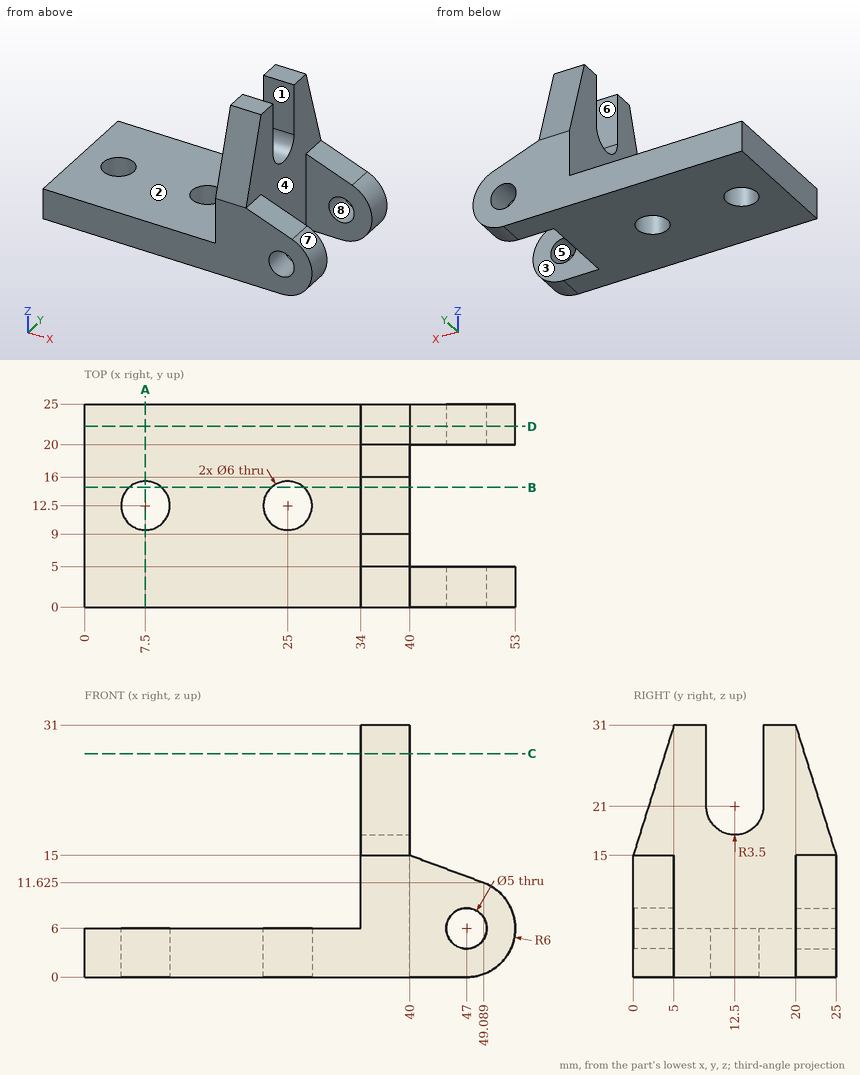
Here's the drawing with two shaded views (mm, measured from the low corner). I have some questions. A direction names the side the tool comes from. Coordinates: 2 decimals unless noted, no trailing zeros. Write each loop counter-clockwise with the first axis right and the second up, starting at its lowest first coordinate (ties: lowest second). Pieces come first, ordered by that corner, then holes.
Item 1: I want a section at A-A on x = 7.5. Write out the boundary of the cut face in (y, z), and give its area (3 significant figures).
Item 2: I want a section at D-D on y = 22.25. Write out the boundary of the cut face in (x, z) (1 decimal).
Item 3: If I drill on line 1 (Y direction, x = 25, z = 3); line 2 (X direction, y = 21.75, z = 22); line 3 (Y direction, x = 5, z = 3), over which ranges is the centre line in solid material (lowest first)?
Item 4: I want a section at B-B on y = 14.75. Write out the boundary of the cut face in (x, z) (1 decimal), and give its area (3 significant figures).
Item 5: I want a section at C-C on z = 27.5. Write out the boundary of the cut face in (x, y).
Item 6: On a 3-axis mill with a long thin cutter (end or side, diameter ignored), from which of +Z, -Z, +X, -X, +Y, -Y can I reach the whole of each face in a straight line? I mean the marked faces 1, 2, 3 and 4. Say none if no direction works.
Item 7: If we mould it in two halves opening along X, with no side actions, what happens to the marked faces 5, 6, 7 and 8? For each: +X half, -X half, draft (parallel to the pull), parting line (faces both ways), or undercut.
Item 8: Will these pins go through, and if not, where does the flat tip stop? pin 1 (3 mm diameter, centred on x = 47, z = 6, fed in from +Y); pin 2 (7.5 mm diameter, centred on x = 14, y = 16, fed in from +Z); pin 3 (1.8 mm diameter, centred on x = 36.5, z = 24, fed in from -Y); pin 4 (12.5 mm diameter, centred on y = 9.5, z = 22, fed in from -X).
Findings below:
1. outline: (0, 0) - (9.5, 0) - (9.5, 6) - (0, 6) - close; (15.5, 0) - (25, 0) - (25, 6) - (15.5, 6) - close
1. area: 114 mm2
2. outline: (0, 0) - (47, 0) arc R6 ccw to (49.1, 11.6) - (40, 15) - (40, 23.8) - (34, 23.8) - (34, 6) - (0, 6) - close; hole circle Ø5 at (47, 6)
3. line 1: y = 0 to 9.5, 15.5 to 25
3. line 2: x = 34 to 40
3. line 3: y = 0 to 10.84, 14.16 to 25
4. outline: (0, 0) - (5.5, 0) - (5.5, 6) - (0, 6) - close; (9.5, 0) - (23, 0) - (23, 6) - (9.5, 6) - close; (27, 0) - (40, 0) - (40, 18.3) - (34, 18.3) - (34, 6) - (27, 6) - close
4. area: 266 mm2
5. outline: (34, 3.91) - (40, 3.91) - (40, 9) - (34, 9) - close; (34, 16) - (40, 16) - (40, 21.09) - (34, 21.09) - close
6. face 1: +Z, +X, -X
6. face 2: +Z, -X, +Y, -Y
6. face 3: +Z, -Z, +X
6. face 4: +Z, +X
7. face 5: undercut
7. face 6: draft
7. face 7: +X half
7. face 8: undercut
8. pin 1: passes through
8. pin 2: stops at z = 6
8. pin 3: stops at y = 2.53
8. pin 4: stops at x = 34
